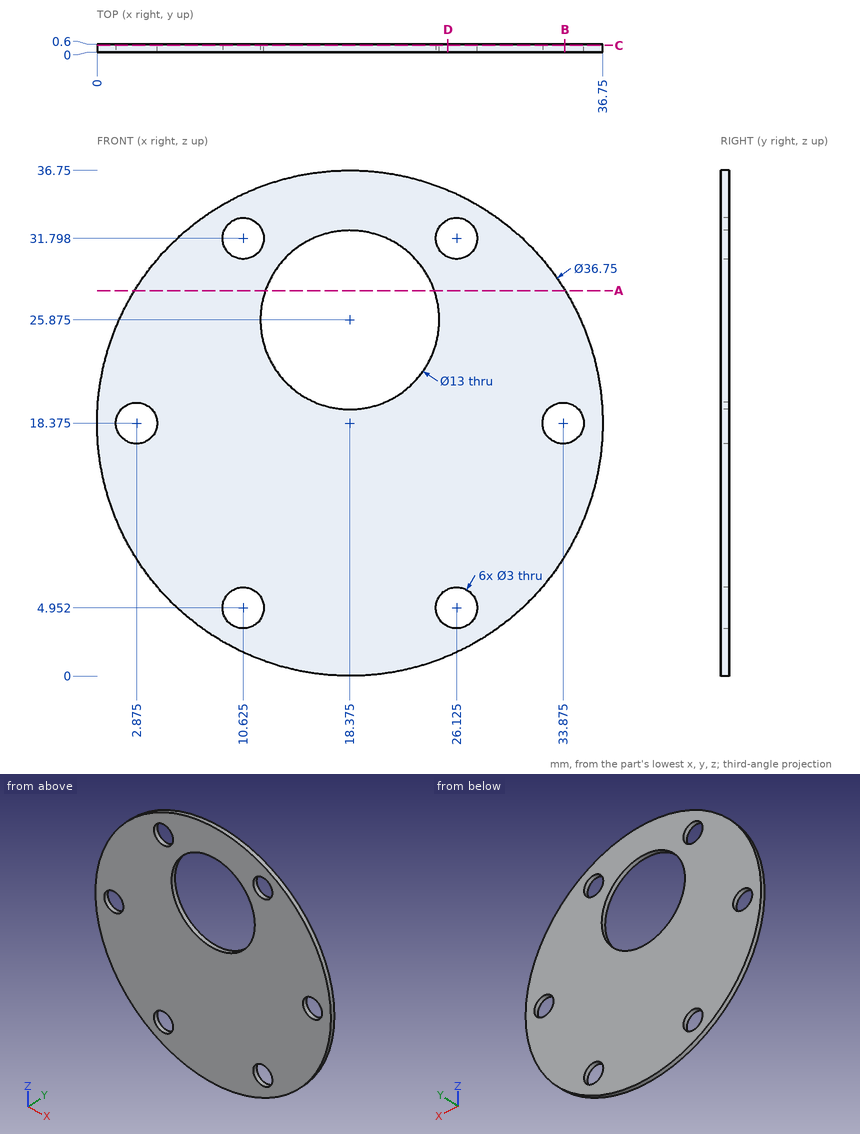
Answer from the drawing. Dimensions are ordinates in mm from the lowest x, y and z of the part. Give positions to 0.01 mm unless a question says otherwise; leave off trailing zeros. Loops run counter-clockwise (first coordinate to the right, second up) from the corner with the lowest first, then second, coordinate; pieces in that order, holes last. Notation, with made-up numbers: (16, 21.25) - (46, 21.25) arc R16 ccw to (46, 39.25) - close; hole circle Ø6 at (32, 89). An arc over 180 degrees is marked (long way). Answer as a JSON object with one key per item and string values.
1. A cutting plane is placed at D-D (x = 25.5). Write down the section's boundary in (y, z) (1 decimal).
Determined:
{"outline": "(0, 1.4) - (0.6, 1.4) - (0.6, 3.6) - (0, 3.6) - close; (0, 6.3) - (0.6, 6.3) - (0.6, 30.4) - (0, 30.4) - close; (0, 33.2) - (0.6, 33.2) - (0.6, 35.3) - (0, 35.3) - close"}
2. A cutting plane is placed at A-A (z = 28). Write down the section's boundary in (x, y).
Determined:
{"outline": "(2.72, 0) - (12.23, 0) - (12.23, 0.6) - (2.72, 0.6) - close; (24.52, 0) - (34.03, 0) - (34.03, 0.6) - (24.52, 0.6) - close"}
3. Find the intervals of material crossed by L1, parallel to X at y = 0.2, z = 5.5 (1 decimal); L2, parallel to Z at x = 11.5, y = 0.5 (1 decimal); L3, parallel to X at y = 0.55, z = 19, in increasing order. Write a range as [from, to].
Determined:
{"L1": "[5.3, 9.2], [12, 24.7], [27.5, 31.5]", "L2": "[1.3, 3.7], [6.2, 30.6], [33, 35.4]", "L3": "[0.01, 1.51], [4.24, 32.51], [35.24, 36.74]"}
4. A cutting plane is placed at C-C (y = 0.5). Give the number of separate pieces and of enclosed holes in the cut face.
Determined:
{"separate pieces": "1", "enclosed holes": "7"}
5. A cutting plane is placed at B-B (x = 34). Write down the section's boundary in (y, z) (1 decimal).
Determined:
{"outline": "(0, 8.7) - (0.6, 8.7) - (0.6, 16.9) - (0, 16.9) - close; (0, 19.9) - (0.6, 19.9) - (0.6, 28) - (0, 28) - close"}
